Print and shaded views of the part. All mm, measured from the part's lowest x, y and z. Coordinates: 2 decimals unless noted, no trailing zeros. Loops run counter-clockwise (first coordinate to the right, second up) from the corner with the lowest first, then second, coordinate; pieces in that order, holes last. Notation, with made-up numbers: (-1, -25.5) -> (29, -25.5) arc R26 ccw to (29, -10.5) -> close; hole circle Ø11 at (65.5, 46). An arc over 180 degrees is marked (long way). One line per question, with ' | ' between items. Start each with the question number.
1) Cut at C-C (z = 10.25). List the corners of the cut face in (x, y), plus the area to 3 significant figures.
2) Probe L1, parallel to Y at x = 2.1, z = 3.5; L2, parallel to Z at x = 0.2, y = 94; L3, parallel to Y at x = 3.2, z = 9.75. List the from-to ranges inside material, lowest first. Write a range as from..to.
3) Drop a flat-ended pin along its axis: pin 1 (2 mm diameter, centred on x = 2, y = 96, fed in from -Z). Give the stop position or say it passes through.
4) Cut at B-B (x = 2.1). List the corners of the cut face in (y, z).
5) Cut at A-A (z = 4). List the corners of the cut face in (x, y).
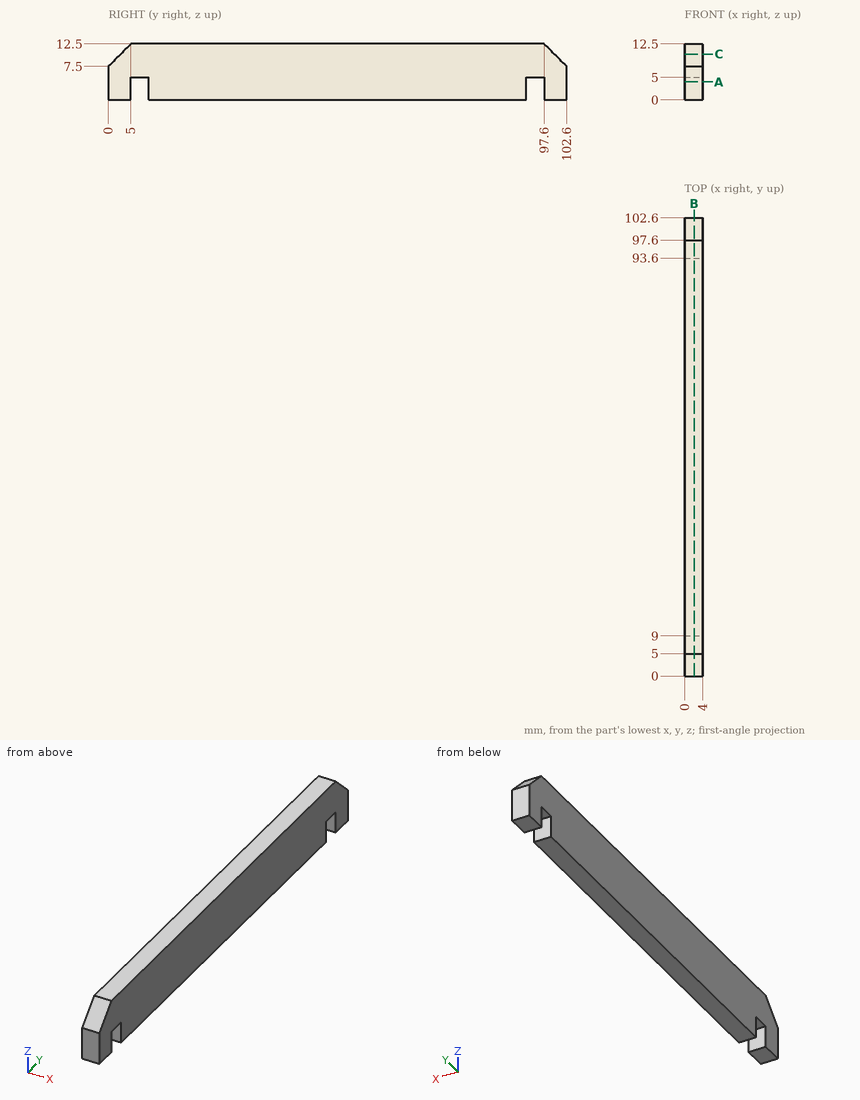
Reported:
1) outline: (0, 2.75) -> (4, 2.75) -> (4, 99.85) -> (0, 99.85) -> close | area: 388 mm²
2) L1: y = 0..5, 9..93.6, 97.6..102.6 | L2: z = 5..12.5 | L3: y = 2.25..100.35
3) pin 1: stops at z = 5
4) outline: (0, 0) -> (5, 0) -> (5, 5) -> (9, 5) -> (9, 0) -> (93.6, 0) -> (93.6, 5) -> (97.6, 5) -> (97.6, 0) -> (102.6, 0) -> (102.6, 7.5) -> (97.6, 12.5) -> (5, 12.5) -> (0, 7.5) -> close
5) outline: (0, 0) -> (4, 0) -> (4, 5) -> (0, 5) -> close; (0, 9) -> (4, 9) -> (4, 93.6) -> (0, 93.6) -> close; (0, 97.6) -> (4, 97.6) -> (4, 102.6) -> (0, 102.6) -> close
